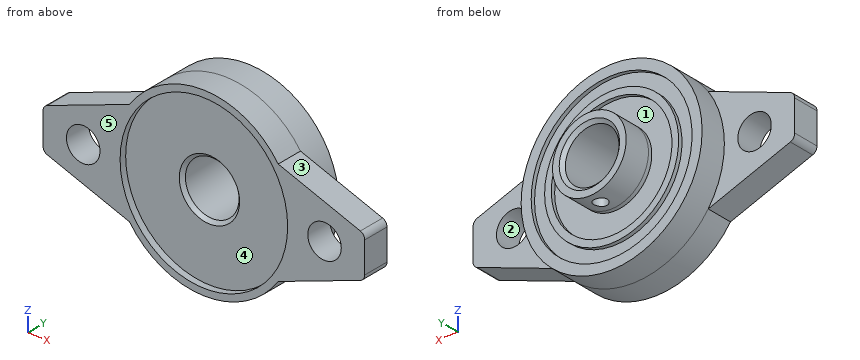
```python
from build123d import *

# Parameters (mm, degrees)
SKETCH_1_R          = 2.5
EXTRUDE_1_DEPTH     = 4
SKETCH_2_R          = 13.5
EXTRUDE_2_DEPTH     = 4
SKETCH_3_R          = 5.5
EXTRUDE_3_DEPTH     = 4
SKETCH_4_R          = 4
CUT_EXTRUDE_1_DEPTH = 13
SKETCH_5_R          = 12
SKETCH_5_R_2        = 10
SKETCH_5_R_3        = 9
SKETCH_5_R_4        = 5.5
CUT_EXTRUDE_2_DEPTH = 0.6
SKETCH_8_R          = 12.5
CUT_EXTRUDE_4_DEPTH = 1
SKETCH_9_R          = 1
CUT_EXTRUDE_5_DEPTH = 14.5
CHAMFER_1_SIZE      = 0.5


with BuildPart() as part:
    # 草图1 → 凸台-拉伸1 (new body)
    with BuildSketch(Plane(origin=(0, 0, 0), x_dir=(1, 0, 0), z_dir=(0, 1, 0))):
        with BuildLine():
            Line((24, -2.299792462), (24, 2.299792462))
            ThreePointArc((24, 2.299792462), (23.819152044, 2.873368898), (23.342020143, 3.239485083))
            Line((23.342020143, 3.239485083), (11.089367754, 7.699085843))
            ThreePointArc((11.089367754, 7.699085843), (0, 13.5), (-11.089367754, 7.699085843))
            Line((-11.089367754, 7.699085843), (-23.342020143, 3.239485083))
            ThreePointArc((-23.342020143, 3.239485083), (-23.819152044, 2.873368898), (-24, 2.299792462))
            Line((-24, 2.299792462), (-24, -2.299792462))
            ThreePointArc((-24, -2.299792462), (-23.819152044, -2.873368898), (-23.342020143, -3.239485083))
            Line((-23.342020143, -3.239485083), (-11.089367754, -7.699085843))
            ThreePointArc((-11.089367754, -7.699085843), (0, -13.5), (11.089367754, -7.699085843))
            Line((11.089367754, -7.699085843), (23.342020143, -3.239485083))
            ThreePointArc((23.342020143, -3.239485083), (23.819152044, -2.873368898), (24, -2.299792462))
        make_face()
        with Locations((-18, 0)):
            Circle(SKETCH_1_R, mode=Mode.SUBTRACT)
        with Locations((18, 0)):
            Circle(SKETCH_1_R, mode=Mode.SUBTRACT)
    extrude(amount=EXTRUDE_1_DEPTH)

    # 草图2 → 凸台-拉伸2 (add)
    with BuildSketch(Plane(origin=(0, 4, 0), x_dir=(1, 0, 0), z_dir=(0, 1, 0))):
        Circle(SKETCH_2_R)
    extrude(amount=EXTRUDE_2_DEPTH)

    # 草图3 → 凸台-拉伸3 (add)
    with BuildSketch(Plane(origin=(0, 8, 0), x_dir=(1, 0, 0), z_dir=(0, 1, 0))):
        Circle(SKETCH_3_R)
    extrude(amount=EXTRUDE_3_DEPTH)

    # 草图4 → 切除-拉伸1 (cut, through all)
    with BuildSketch(Plane(origin=(0, 12, 0), x_dir=(1, 0, 0), z_dir=(0, 1, 0))):
        Circle(SKETCH_4_R)
    extrude(amount=-CUT_EXTRUDE_1_DEPTH, mode=Mode.SUBTRACT)

    # 草图5 → 切除-拉伸2 (cut)
    with BuildSketch(Plane(origin=(0, 8, 0), x_dir=(1, 0, 0), z_dir=(0, 1, 0))):
        Circle(SKETCH_5_R)
        Circle(SKETCH_5_R_2, mode=Mode.SUBTRACT)
        Circle(SKETCH_5_R_3)
        Circle(SKETCH_5_R_4, mode=Mode.SUBTRACT)
    extrude(amount=-CUT_EXTRUDE_2_DEPTH, mode=Mode.SUBTRACT)

    # 草图8 → 切除-拉伸4 (cut)
    with BuildSketch(Plane.XZ):
        Circle(SKETCH_8_R)
    extrude(amount=-CUT_EXTRUDE_4_DEPTH, mode=Mode.SUBTRACT)

    # 草图9 → 切除-拉伸5 (cut, through all)
    with BuildSketch(Plane.XY):
        with Locations((0, 10)):
            Circle(SKETCH_9_R)
    extrude(amount=-CUT_EXTRUDE_5_DEPTH, mode=Mode.SUBTRACT)

    # 倒角1
    chamfer_1_edges = [part.edges().sort_by_distance(p)[0] for p in [
        (-4, 12, 0),
        (-4, 1, 0),
    ]]
    chamfer(chamfer_1_edges, length=CHAMFER_1_SIZE)


solid = part.part
```
Here's how the part is built. I have some questions about the finished solid (model axes, mm). Face numbers are marked on the shaded views. A direction names the side the tool comes from. Coordinates: 2 decimals unless noted, no trailing zeros. Order: outer loops, then holes, each group sorted by start corner. A loop starts at its lowest first (then second) coordinate and runs counter-clockwise, first axis right, second up. Notation, with made-up numbers: M 49.25,13.5 L 63.25,13.5 A29 ccw 63.25,40.5 Z; hole C 80.25,-12 d4. An arc over 180 degrees is marked long. Answer as a JSON object with one key per item and string values. Group by question number.
(1) Suppose I cut it at B-B, the plane x = -18. Please give me the cut outline in (y, z), then the cut area to 3 significant figures.
(2) Which directions (+Z, -Z, +X, -X, +Y, -Y) give clear straight access to the entire face, cutting with the end or side of a thin tool? Please do the marked faces 1 and 2.
(3) Suppose I cut it at A-A, the plane y = 3. Please give me the cut outline in (x, z).
(4) Suppose I cut it at C-C, the plane y = 5.25. Please give me the cut outline in (x, z), then the cut area to 3 significant figures.
(5) If we mould it in two halves opening along Z, with no side actions, what happens to the marked faces 3, 4 and 5? For each: released by +Z, released by -Z, zero draft, split by the parting line, or undercut.
(6) Suppose I cut it at D-D, the plane z = 0. State how many separate pieces and enclosed holes the cut face has, then the cut area to 3 significant figures.
(7) I need wall thicknesses on probe 1 along X at (y, z) = (2.95, 0); probe 2 along Y at (x, z) = (0, -4.7); probe 3 along Z at (x, y) = (0, 0.8). Which ranges of each line are inside material? Lowest first, please.
(8) For pin 1 (1 mm diameter, centred on x = 7, y = 8, fed in from +Z); pin 2 (4.5 mm diameter, centred on x = 18, z = 0, fed in from -Y); pin 3 (1.5 mm diameter, centred on x = -9, z = 6, fed in from +Y); pin 4 (10.5 mm diameter, centred on x = 16.5, z = 3.5, fed in from +Y), each with a flat end and sliding along its axis, tell me the tip position at first contact or that it passes through.
Values found:
{
 "1": {"outline": "M 0,-5.18 L 4,-5.18 L 4,-2.5 L 0,-2.5 Z; M 0,2.5 L 4,2.5 L 4,5.18 L 0,5.18 Z", "area": "21.5 mm^2"},
 "2": {"face 1": "+Y", "face 2": "+Y, -Y"},
 "3": {"outline": "M -24,-2.3 A1 ccw -23.34,-3.24 L -11.09,-7.7 A13.5 ccw 11.09,-7.7 L 23.34,-3.24 A1 ccw 24,-2.3 L 24,2.3 A1 ccw 23.34,3.24 L 11.09,7.7 A13.5 ccw -11.09,7.7 L -23.34,3.24 A1 ccw -24,2.3 Z; hole C -18,0 d5; hole C 0,0 d8; hole C 18,0 d5"},
 "4": {"outline": "C 0,0 d27; hole C 0,0 d8", "area": "522 mm^2"},
 "5": {"face 3": "released by +Z", "face 4": "undercut", "face 5": "zero draft"},
 "6": {"separate pieces": "4", "enclosed holes": "0", "area": "184 mm^2"},
 "7": {"probe 1": "x = -24 to -20.5, -15.5 to -4, 4 to 15.5, 20.5 to 24", "probe 2": "y = 1 to 9, 11 to 12", "probe 3": "z = -13.5 to -12.5, 12.5 to 13.5"},
 "8": {"pin 1": "stops at z = 11.83", "pin 2": "passes through", "pin 3": "stops at y = 7.4", "pin 4": "stops at y = 8"}
}
